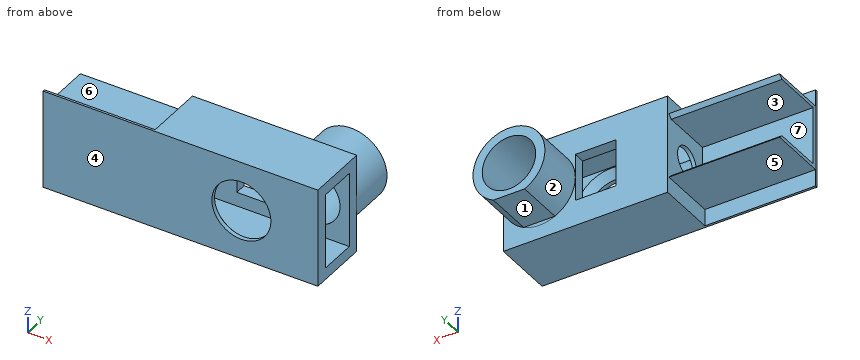
from build123d import *

# Parameters (mm, degrees)
SKETCH2_W            = 26.8
SKETCH2_H            = 16.6
SKETCH2_W_2          = 20.8
SKETCH2_H_2          = 10.6
BOSS_EXTRUDE3_DEPTH  = 19.5
SKETCH8_R            = 9.75
SKETCH8_R_2          = 7.25
BOSS_EXTRUDE5_DEPTH  = 13.010482488
CUT_EXTRUDE1_START   = -5
SKETCH9_R            = 7.25
CUT_EXTRUDE1_DEPTH   = 5
SKETCH11_W           = 20.8
SKETCH11_H           = 10.6
SKETCH11_W_2         = 20.4
SKETCH11_H_2         = 10.3
BOSS_EXTRUDE7_DEPTH  = 19.5
SKETCH12_R           = 7.248274147
CUT_EXTRUDE3_DEPTH   = 4
SKETCH14_W           = 26.8
SKETCH14_H           = 16.6
SKETCH14_W_2         = 20.4
SKETCH14_H_2         = 10.3
BOSS_EXTRUDE8_DEPTH  = 24
SKETCH15_R           = 8
CUT_EXTRUDE5_DEPTH   = 5
SKETCH16_W           = 11.004107939
SKETCH16_H           = 12.8
CUT_EXTRUDE6_DEPTH   = 5
CHAMFER4_SIZE        = 2
SKETCH17_W           = 26.8
SKETCH17_H           = 16.6
BOSS_EXTRUDE9_DEPTH  = 1
SKETCH18_R           = 4
CUT_EXTRUDE7_DEPTH   = 1
BOSS_EXTRUDE11_DEPTH = 30
SKETCH20_W           = 30.011261772
SKETCH20_H           = 26.8
BOSS_EXTRUDE12_DEPTH = 0.6
SKETCH23_R           = 6.70324332
CUT_EXTRUDE9_DEPTH   = 5
SKETCH25_W           = 20.840121468
SKETCH25_H           = 2.448199345
CUT_EXTRUDE10_DEPTH  = 13.01


with BuildPart() as part:
    # Sketch2 → Boss-Extrude3 (new body)
    with BuildSketch(Plane(origin=(0, 0, 0), x_dir=(0, 0, -1), z_dir=(1, 0, 0))):
        with Locations((9.011494253, 5.445783842)):
            Rectangle(SKETCH2_W, SKETCH2_H)
        with Locations((9.011494253, 5.445783842)):
            Rectangle(SKETCH2_W_2, SKETCH2_H_2, mode=Mode.SUBTRACT)
    extrude(amount=BOSS_EXTRUDE3_DEPTH)

    # Sketch8 → Boss-Extrude5 (add)
    with BuildSketch(Plane(origin=(0, 13.745783842, 0), x_dir=(1, 0, 0), z_dir=(0, 1, 0))):
        with Locations(Location((9.75, 9.011494253, 0), (0, 0, 180))):
            Circle(SKETCH8_R)
        with Locations(Location((9.75, 9.011494253, 0), (0, 0, 270))):
            Circle(SKETCH8_R_2, mode=Mode.SUBTRACT)
    extrude(amount=BOSS_EXTRUDE5_DEPTH)

    # Sketch9 → Cut-Extrude1 (cut)
    with BuildSketch(Plane(origin=(0, 13.745783842, 0), x_dir=(1, 0, 0), z_dir=(0, 1, 0)).offset(CUT_EXTRUDE1_START)):
        with Locations(Location((9.75, 9.011494253, 0), (0, 0, 270))):
            Circle(SKETCH9_R)
    extrude(amount=CUT_EXTRUDE1_DEPTH, mode=Mode.SUBTRACT)

    # Sketch11 → Boss-Extrude7 (add)
    with BuildSketch(Plane.ZY):
        with Locations((-9.011494253, 5.445783842)):
            Rectangle(SKETCH11_W, SKETCH11_H)
        with Locations((-9.011494253, 5.445783842)):
            Rectangle(SKETCH11_W_2, SKETCH11_H_2, mode=Mode.SUBTRACT)
    extrude(amount=-BOSS_EXTRUDE7_DEPTH)

    # Sketch12 → Cut-Extrude3 (cut)
    with BuildSketch(Plane(origin=(0, 13.745783842, 0), x_dir=(1, 0, 0), z_dir=(0, 1, 0))):
        with Locations(Location((9.75, 9.011494253, 0), (0, 0, 270))):
            Circle(SKETCH12_R)
    extrude(amount=-CUT_EXTRUDE3_DEPTH, mode=Mode.SUBTRACT)

    # Sketch14 → Boss-Extrude8 (add)
    with BuildSketch(Plane.ZY):
        with Locations((-9.011494253, 5.445783842)):
            Rectangle(SKETCH14_W, SKETCH14_H)
        with Locations((-9.011494253, 5.445783842)):
            Rectangle(SKETCH14_W_2, SKETCH14_H_2, mode=Mode.SUBTRACT)
    extrude(amount=BOSS_EXTRUDE8_DEPTH)

    # Sketch15 → Cut-Extrude5 (cut)
    with BuildSketch(Plane.XZ.offset(2.854216158)):
        with Locations(Location((-1.242459593, -9.011494253, 0), (0, 0, 270))):
            Circle(SKETCH15_R)
    extrude(amount=-CUT_EXTRUDE5_DEPTH, mode=Mode.SUBTRACT)

    # Sketch16 → Cut-Extrude6 (cut)
    with BuildSketch(Plane(origin=(0, 13.745783842, 0), x_dir=(1, 0, 0), z_dir=(0, 1, 0))):
        with Locations((-5.50205397, 9.011494253)):
            Rectangle(SKETCH16_W, SKETCH16_H)
    extrude(amount=-CUT_EXTRUDE6_DEPTH, mode=Mode.SUBTRACT)

    # Chamfer4
    chamfer4_edges = [part.edges().sort_by_distance(p)[0] for p in [
        (-1.242459593, 0.295783842, -1.011494253),
    ]]
    chamfer(chamfer4_edges, length=CHAMFER4_SIZE)

    # Sketch17 → Boss-Extrude9 (add)
    with BuildSketch(Plane.ZY.offset(24)):
        with Locations((-9.011494253, 5.445783842)):
            Rectangle(SKETCH17_W, SKETCH17_H)
    extrude(amount=BOSS_EXTRUDE9_DEPTH)

    # Sketch18 → Cut-Extrude7 (cut)
    with BuildSketch(Plane.ZY.offset(25)):
        with Locations((-9.011494253, 5.445783842)):
            Circle(SKETCH18_R)
    extrude(amount=-CUT_EXTRUDE7_DEPTH, mode=Mode.SUBTRACT)

    # Sketch19 → Boss-Extrude11 (add)
    with BuildSketch(Plane.ZY.offset(25)):
        Polygon((-0.161494253, 13.145783842), (-0.161494253, -2.254216158), (-17.861494253, -2.254216158), (-17.861494253, 13.145783842), (-16.861494253, 12.145783842), (-16.861494253, -1.254216158), (-1.161494253, -1.254216158), (-1.161494253, 12.145783842), align=None)
    extrude(amount=BOSS_EXTRUDE11_DEPTH)

    # Sketch20 → Boss-Extrude12 (add)
    with BuildSketch(Plane.XZ.offset(2.254216158)):
        with Locations((-40.005630886, -9.011494253)):
            Rectangle(SKETCH20_W, SKETCH20_H)
    extrude(amount=BOSS_EXTRUDE12_DEPTH)

    # Sketch23 → Cut-Extrude9 (cut)
    with BuildSketch(Plane(origin=(-24, 0, 0), x_dir=(0, 0, -1), z_dir=(1, 0, 0))):
        with Locations((9.011494253, 5.445783842)):
            Circle(SKETCH23_R)
    extrude(amount=CUT_EXTRUDE9_DEPTH, mode=Mode.SUBTRACT)

    # Sketch25 → Cut-Extrude10 (cut)
    with BuildSketch(Plane(origin=(0, 26.756266329, 0), x_dir=(1, 0, 0), z_dir=(0, 1, 0))):
        with Locations((10.420060734, 19.018301842)):
            Rectangle(SKETCH25_W, SKETCH25_H)
    extrude(amount=-CUT_EXTRUDE10_DEPTH, mode=Mode.SUBTRACT)


solid = part.part
For this review, take the finished solid that the model builds, in its own axes (mm). Face numbers are marked on the shaded views. A direction names the side the tool comes from. Round coordinates to 2 decimals unless told otherwise and drop trailing zeros. Loops run counter-clockwise (first coordinate to the right, second up) from the corner with the lowest first, then second, coordinate; pieces in that order, holes last. Notation, with made-up numbers: (80.5, 15.25) - (122.5, 15.25) arc R14 cw to (122.5, 40.25) - close; hole circle Ø1 at (45, 34). An arc over 180 degrees is marked (long way). One line per item, written item: value. Start each with the question number.
Item 1: For L1, parallel to X at y = 20.5, z = -8.5; L2, parallel to Y at x = -19.5, z = -13.75; L3, parallel to Z at x = 9.75, y = 21, list the stretches that pass through material, from the lowest coordinate up.
Item 2: Take a section at D-D (z = -10.5). State how many separate pieces and enclosed holes the cut face has, plus the area to 3 significant figures.
Item 3: For the marked faces 5, 6 and 7, list the 3-axis set-ups (+Z, -Z, +X, -X, +Y, -Y) from which the entire face can be reached by the end or side of a thin tool; tool diameter is ignored.
Item 4: Take a section at A-A (x = -21.5). Give the boundary of the cut face in (y, z).
Item 5: Take a section at C-C (y = 21.25). Give the boundary of the cut face in (x, z).
Item 6: The part is to be moulded in two halves that separate along Z. For the marked faces 1, 2, 3 and 4, say which applies: +Z half, -Z half, draft (parallel to the pull), parting line (faces both ways), or undercut.
Item 7: Clearance check with flat-ended pins moving along their axes: pin 1 Ø8 at (x, z) = (-25, -8.5) entering from +Y; pin 2 Ø5 at (y, z) = (16, -5) entering from -X; pin 3 Ø7 at (x, z) = (11.5, -11.5) entering from +Y; pin 4 Ø1.5 at (x, y) = (-32.5, 15) entering from +Z. State where each tip first meets the part, or that it passes through.
Item 8: Take a section at B-B (x = -36). Give the boundary of the cut face in (y, z), plus the area to 3 significant figures.
Answer below:
1. L1: x = 0.01 to 2.52, 16.98 to 19.49
1. L2: y = -2.85 to 0.3, 10.6 to 13.75
1. L3: z = -17.79 to -16.26, -1.76 to 0.74
2. separate pieces: 5
2. enclosed holes: 0
2. area: 251 mm2
3. face 5: -Z, -X, +Y
3. face 6: +Z, -X, +Y
3. face 7: -X, +Y
4. outline: (-2.85, -22.41) - (13.75, -22.41) - (13.75, 4.39) - (-2.85, 4.39) - close; hole (0.3, -19.21) - (10.6, -19.21) - (10.6, -13.3) arc R6.7 ccw to (10.6, -4.72) - (10.6, 1.19) - (0.3, 1.19) - (0.3, -4.72) arc R6.7 ccw to (0.3, -13.3) - close
5. outline: (5.52, -17.79) - (13.98, -17.79) arc R9.75 ccw (long way) to start; hole circle Ø14.5 at (9.75, -9.01)
6. face 1: -Z half
6. face 2: parting line
6. face 3: undercut
6. face 4: draft
7. pin 1: stops at y = 13.75
7. pin 2: stops at x = -25
7. pin 3: stops at y = 0.3
7. pin 4: passes through
8. outline: (-2.85, -22.41) - (-2.25, -22.41) - (-2.25, -17.86) - (13.15, -17.86) - (12.15, -16.86) - (-1.25, -16.86) - (-1.25, -1.16) - (12.15, -1.16) - (13.15, -0.16) - (-2.25, -0.16) - (-2.25, 4.39) - (-2.85, 4.39) - close
8. area: 61.6 mm2
